Check sheet for the modelled part. Datum: model origin and axes. Units: mm. A direction names the side the tool comes from. Give positions to 0.01 mm unless a question says otherwise; leave off trailing zeros. Write each loop counter-clockwise with the first axis right and the second up, starting at its lowest first coordinate (ties: lowest second). Pieces come first, ordered by that corner, then holes. Notation, with made-up numbers: (-14.75, -23) -> (13.25, -23) arc R20 ccw to (13.25, 4) -> close; hole circle Ø7 at (16.25, 18). An arc over 180 degrees is marked (long way). Use a Markdown table: item, result. Add a question column.
1. Gauge pin test, flat ends, axial feed: P1, Ø1.5, axis at x = 4, y = -4, coming from the +Z side; P2, Ø5, axis at x = 5, z = -0.5, coming from the -Y side; P3, Ø2.5, axis at x = 5, y = -4.5, coming from the -Z side. Record the tip position at first contact, or that the pin passes through.
2. Cross-section at C-C (z = -12.5). Enter the section's corners in (x, y).
3. Cross-section at B-B (y = -12). Enter the section's corners in (x, z).
4. Release check for a two-part mould opening along Y. For faces 1 (the cylindrical face through (5.916, 13.318, 1.212)), 2 (the cylindrical face through (5.916, -12.1, -5.694)), 3 (the cylindrical face through (5.916, 1.119, 13.326)) record: released by +Y, released by -Y, zero draft, split by the parting line, or undercut.
5. Cross-section at A-A (z = 0). Enter the section's corners in (x, y), then the cut area to 3 significant figures.
6. Set-up check for faces 4 (the cylindrical face through (5.916, 3.506, -12.905)), 5 (the cylindrical face through (5.916, 11.03, 7.645)), 6 (the cylindrical face through (5.92, -13.36, 1.23)), 7 (the cylindrical face through (5.916, -3.506, 12.905)): record each of +Z, -Z, +X, -X, +Y, -Y from which the full face is reachable in a straight line by a thin tool's end or side.
7. Scan lines: probe 1 along Y at (x, z) = (2.25, -12.75); probe 2 along Y at (x, z) = (1, -2.25); probe 3 along Y at (x, z) = (7.5, 11). Record each from-to range of solid material in increasing order. Write a range as [from, to].
8. Cross-section at D-D (y = 1.75). Enter the section's corners in (x, z), then the cut area to 3 significant figures.
from build123d import *

# Parameters (mm, degrees)
BASPROSKE_W        = 12
BASPROSKE_H        = 15
TOOTHCUT_DEPTH     = 25.372115214
TEETHCUTS_COUNT    = 18
TEETHCUTS_ANGLE    = 340
BORSKE_R           = 2
BORE_DEPTH         = 50.0000508
SKETCH2_W          = 3
SKETCH2_H          = 6
SKETCH2_W_2        = 6
SKETCH2_H_2        = 3
CUT_EXTRUDE2_DEPTH = 16


with BuildPart() as part:
    # BasProSke → Base-Revolve (revolve)
    with BuildSketch(Plane(origin=(0, 0, 0), x_dir=(1, 0, 0), z_dir=(0, 1, 0)), mode=Mode.PRIVATE) as base_revolve_sk:
        with Locations((6, 7.5)):
            Rectangle(BASPROSKE_W, BASPROSKE_H)
    revolve(base_revolve_sk.sketch.rotate(Axis((-10, 0, 0), (1, 0, 0)), 180), axis=Axis((-10, 0, 0), (1, 0, 0)))

    # TooCutSke → ToothCut (cut, through all)
    with BuildSketch(Plane(origin=(0, 0, 0), x_dir=(0, 0, -1), z_dir=(1, 0, 0))):
        with BuildLine():
            ThreePointArc((0.759974923, 11.599129886), (0, 11.624), (-0.759974923, 11.599129886))
            ThreePointArc((-0.759974923, 11.599129886), (-1.229186471, 13.354767823), (-2.254227748, 14.855339189))
            ThreePointArc((-2.254227748, 14.855339189), (0, 15.0254), (2.254227748, 14.855339189))
            ThreePointArc((2.254227748, 14.855339189), (1.229186471, 13.354767823), (0.759974923, 11.599129886))
        make_face()
    toothcut = extrude(amount=TOOTHCUT_DEPTH, mode=Mode.SUBTRACT)

    # TeethCuts: ToothCut ×18 about axis
    teethcuts_axis = Axis((-10, 0, 0), (1, 0, 0))
    for i in range(1, TEETHCUTS_COUNT):
        add(toothcut.rotate(teethcuts_axis, i * TEETHCUTS_ANGLE / (TEETHCUTS_COUNT - 1)), mode=Mode.SUBTRACT)

    # BorSke → Bore (cut, symmetric)
    with BuildSketch(Plane(origin=(0, 0, 0), x_dir=(0, 0, -1), z_dir=(1, 0, 0))):
        with Locations(Location((0, 0, 0), (0, 0, 180))):
            Circle(BORSKE_R)
    extrude(amount=BORE_DEPTH, both=True, mode=Mode.SUBTRACT)

    # Sketch2 → Cut-Extrude2 (cut)
    with BuildSketch(Plane(origin=(12, 0, 0), x_dir=(0, 0, -1), z_dir=(1, 0, 0))):
        with Locations((-4.5, 0)):
            Rectangle(SKETCH2_W, SKETCH2_H)
        with Locations((0, 4.5)):
            Rectangle(SKETCH2_W_2, SKETCH2_H_2)
        Rectangle(SKETCH2_W_2, SKETCH2_H)
        with Locations((4.5, 0)):
            Rectangle(SKETCH2_W, SKETCH2_H)
        with Locations((0, -4.5)):
            Rectangle(SKETCH2_W_2, SKETCH2_H_2)
    extrude(amount=-CUT_EXTRUDE2_DEPTH, mode=Mode.SUBTRACT)


solid = part.part
Worked answers:
| question | item | result |
|---|---|---|
| 1 | P1 | stops at z = 14.2 |
| 1 | P2 | stops at y = -14.83 |
| 1 | P3 | stops at z = -14.22 |
| 2 | outline | (0, -5.63) -> (12, -5.63) -> (12, -3.26) -> (0, -3.26) -> close; (0, -1.26) -> (12, -1.26) -> (12, 1.26) -> (0, 1.26) -> close; (0, 3.26) -> (12, 3.26) -> (12, 5.63) -> (0, 5.63) -> close |
| 3 | outline | (0, -7.82) -> (12, -7.82) -> (12, -5.6) -> (0, -5.6) -> close; (0, -3.4) -> (12, -3.4) -> (12, -0.81) -> (0, -0.81) -> close; (0, 0.81) -> (12, 0.81) -> (12, 3.4) -> (0, 3.4) -> close; (0, 5.6) -> (12, 5.6) -> (12, 7.82) -> (0, 7.82) -> close |
| 4 | face 1 | released by +Y |
| 4 | face 2 | released by -Y |
| 4 | face 3 | undercut |
| 5 | outline | (0, -11.62) -> (12, -11.62) -> (12, -6) -> (0, -6) -> close; (0, 6) -> (12, 6) -> (12, 11.62) -> (0, 11.62) -> close |
| 5 | area | 135 mm² |
| 6 | face 4 | -Z, +X, -X |
| 6 | face 5 | +X, -X |
| 6 | face 6 | +X, -X, -Y |
| 6 | face 7 | +Z, +X, -X |
| 7 | probe 1 | y = [-5.64, -3.41], [-1.23, 1.23], [3.41, 5.64] |
| 7 | probe 2 | y = [-14.83, -6], [6, 14.83] |
| 7 | probe 3 | y = [-9.89, -7.81], [-5.37, 5.37], [7.81, 9.89] |
| 8 | outline | (0, -11.49) -> (12, -11.49) -> (12, -6) -> (0, -6) -> close; (0, 6) -> (12, 6) -> (12, 11.49) -> (0, 11.49) -> close |
| 8 | area | 132 mm² |
